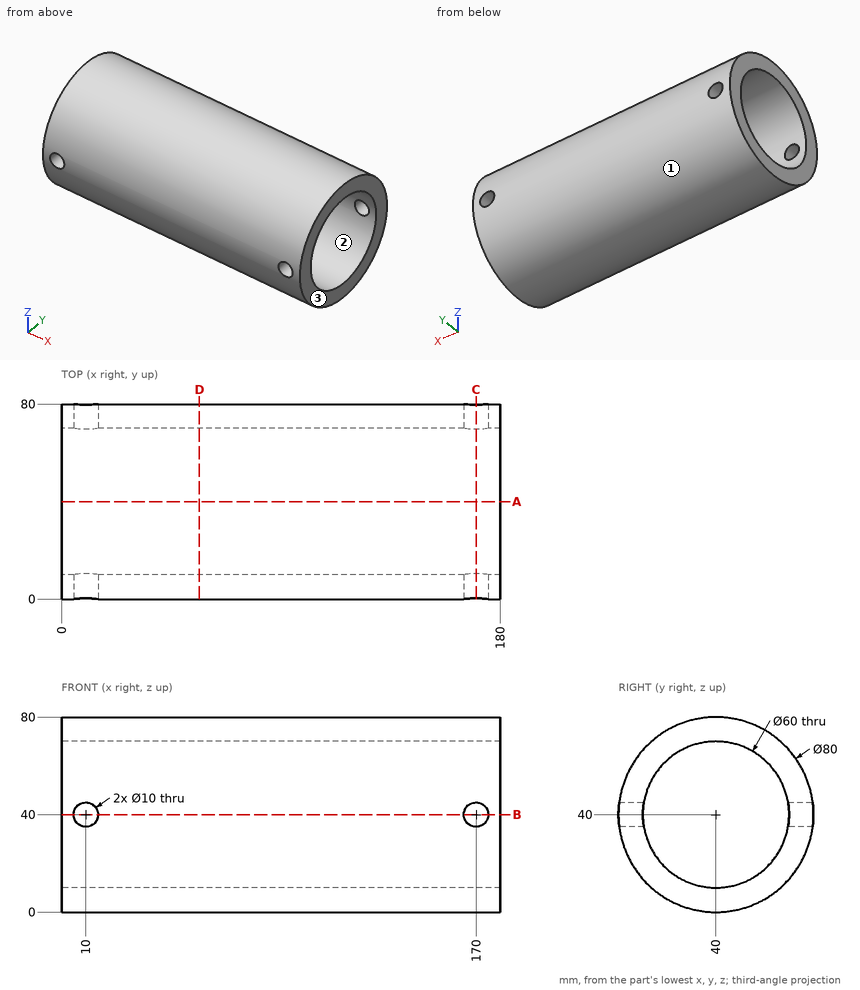
Geometry: see drawing. Coordinates: mm, zero at the bounding-box minimum. Give positions to 0.01 mm unless a question says otherwise; leave off trailing zeros. Order: outer loops, then holes, each group sorted by start corner. A loop starts at its lowest first (then second) coordinate and runs counter-clockwise, first axis right, second up. Notation, with made-up numbers: (77, 40.5) - (126, 40.5) arc R30 cw to (126, 70.5) - close; hole circle Ø2 at (-9, -25.75). An arc over 180 degrees is marked (long way). One line per item, written item: value.
1. Cut plane B-B, the plane z = 40. Output: boundary loops of the cut face in (x, y).
Determined:
outline: (0, 0) - (5, 0) - (5, 10) - (0, 10) - close; (0, 70) - (5, 70) - (5, 80) - (0, 80) - close; (15, 0) - (165, 0) - (165, 10) - (15, 10) - close; (15, 70) - (165, 70) - (165, 80) - (15, 80) - close; (175, 0) - (180, 0) - (180, 10) - (175, 10) - close; (175, 70) - (180, 70) - (180, 80) - (175, 80) - close
2. Cut plane D-D, the plane x = 56.5. Output: boundary loops of the cut face in (y, z), and give its area (3 significant figures).
Determined:
outline: circle Ø80 at (40, 40); hole circle Ø60 at (40, 40)
area: 2,200 mm2
3. Line query: probe 1 along X at (y, z) = (5.25, 40); probe 2 along Z at (x, y) = (111, 39); probe 3 along Y at (x, z) = (43, 40). Output: solid intervals per line, ascending.
Determined:
probe 1: 0 to 5, 15 to 165, 175 to 180
probe 2: 0.01 to 10.02, 69.98 to 79.99
probe 3: 0 to 10, 70 to 80
4. Cut plane C-C, the plane x = 170. Output: boundary loops of the cut face in (y, z), and give its area (3 significant figures).
Determined:
outline: (0.31, 35) arc R40 ccw to (79.69, 35) - (69.58, 35) arc R30 cw to (10.42, 35) - close; (0.31, 45) - (10.42, 45) arc R30 cw to (69.58, 45) - (79.69, 45) arc R40 ccw to start
area: 2,000 mm2
5. Cut plane A-A, the plane y = 40. Output: boundary loops of the cut face in (x, z), and give its area (3 significant figures).
Determined:
outline: (0, 0) - (180, 0) - (180, 10) - (0, 10) - close; (0, 70) - (180, 70) - (180, 80) - (0, 80) - close
area: 3,600 mm2
6. Draft query along Y for the marked faces 1, 2 and 3. Return one class per face: released by +Y, released by -Y, zero draft, split by the parting line, or undercut.
Determined:
face 1: split by the parting line
face 2: undercut
face 3: zero draft
7. Pin query (flat end, axial travel): pin 1 Ø4 at (x, y) = (93.5, 69) entering from -Z; pin 2 Ø1 at (x, z) = (154, 56.5) entering from +Y; pin 3 Ø6 at (x, z) = (40, 70) entering from -Y. Return the tip coordinate at first contact, or that it passes through.
Determined:
pin 1: z = 10.49
pin 2: y = 76.66
pin 3: y = 10.49
